Geometry check sheet. Reference: the model listing, model coordinates, mm. A direction names the side the tool comes from. Give positions to 0.01 mm unless a question says otherwise; leave off trailing zeros. One line per item, written item: value.
from build123d import *

# Parameters (mm, degrees)
SKETCH1_W           = 57.15
SKETCH1_H           = 76.2
BOSS_EXTRUDE1_DEPTH = 3.175
CUT_EXTRUDE1_DEPTH  = 1.27


with BuildPart() as part:
    # Sketch1 → Boss-Extrude1 (new body)
    with BuildSketch(Plane(origin=(0, 0, 0), x_dir=(1, 0, 0), z_dir=(0, 1, 0))):
        Rectangle(SKETCH1_W, SKETCH1_H)
    extrude(amount=BOSS_EXTRUDE1_DEPTH)

    # Sketch2 → Cut-Extrude1 (cut)
    # profile 1 of 4: a face of its own
    with BuildSketch(Plane(origin=(0, 3.175, 0), x_dir=(-1, 0, 0), z_dir=(0, 1, 0))):
        with BuildLine():
            Line((6.055318585, -16.590002596), (5.770382688, -16.590002596))
            Line((5.770382688, -16.590002596), (5.770382688, -16.171502996))
            add(Edge.make_bspline(
                [(5.770382688, -16.171502996), (5.740011779, -16.209517079), (5.68116854, -16.283168869), (5.58216602, -16.379210072), (5.478935847, -16.459804005), (5.3698014, -16.523260139), (5.255885696, -16.571252171), (5.137511969, -16.605860082), (5.01403952, -16.626623661), (4.930069938, -16.629335713), (4.88759022, -16.630707724)],
                knots=[0, 0, 0, 0, 1.127869841, 2.185233117, 3.191641716, 4.159226741, 5.10472073, 6.052603964, 7.014823782, 8, 8, 8, 8], degree=3))
            add(Edge.make_bspline(
                [(4.88759022, -16.630707724), (4.844634079, -16.629214017), (4.760516404, -16.626289008), (4.638482352, -16.600515848), (4.523708355, -16.559729658), (4.417729129, -16.502406678), (4.322175382, -16.431236503), (4.239313996, -16.347753357), (4.169631782, -16.252962996), (4.123122139, -16.164236993), (4.093040195, -16.085425579), (4.073271524, -16.0180161), (4.057278247, -15.942883297), (4.04294765, -15.86021293), (4.033387568, -15.769672957), (4.025809426, -15.671479471), (4.020388991, -15.565649476), (4.020173366, -15.492455289), (4.020062175, -15.454711129)],
                knots=[0, 0, 0, 0, 1.235764162, 2.419900973, 3.574701258, 4.732869372, 5.875730734, 6.993815468, 8.107424371, 9.251605764, 9.866123335, 10.534503958, 11.272175692, 12.077112099, 12.949509943, 13.89253218, 14.913238789, 16, 16, 16, 16], degree=3))
            Line((4.020062175, -15.454711129), (4.020062175, -14.269810288))
            Line((4.020062175, -14.269810288), (4.304998072, -14.269810288))
            Line((4.304998072, -14.269810288), (4.304998072, -15.361216538))
            add(Edge.make_bspline(
                [(4.304998072, -15.361216538), (4.305172614, -15.392805516), (4.305506484, -15.453229854), (4.306573304, -15.539742593), (4.30908455, -15.617988608), (4.312758395, -15.688192769), (4.31790085, -15.750098127), (4.323405942, -15.804018032), (4.330082808, -15.849474875), (4.33603676, -15.876838879), (4.338707007, -15.889111169)],
                knots=[0, 0, 0, 0, 1.430803381, 2.736883362, 3.918614142, 4.976458302, 5.92063272, 6.731858525, 7.431260095, 8, 8, 8, 8], degree=3))
            add(Edge.make_bspline(
                [(4.338707007, -15.889111169), (4.348298036, -15.925160767), (4.366708706, -15.994360559), (4.413127221, -16.088064198), (4.470383963, -16.168488135), (4.541323753, -16.233978346), (4.624041324, -16.28496079), (4.718674187, -16.320307963), (4.824242938, -16.342422975), (4.898497037, -16.344624403), (4.937199595, -16.345771826)],
                knots=[0, 0, 0, 0, 1.084232, 2.08126119, 3.027460722, 3.945137793, 4.874029258, 5.839697328, 6.874011781, 8, 8, 8, 8], degree=3))
            add(Edge.make_bspline(
                [(4.937199595, -16.345771826), (4.960123112, -16.345346396), (5.005488159, -16.344504481), (5.072721891, -16.335837862), (5.13814421, -16.32215003), (5.201579846, -16.301932164), (5.263156997, -16.277350064), (5.323130484, -16.247186672), (5.380662305, -16.210701491), (5.436561438, -16.1696921), (5.488517318, -16.124022995), (5.537550393, -16.076530302), (5.580632017, -16.025225386), (5.619738091, -15.971922216), (5.653454407, -15.915550043), (5.682896587, -15.856711455), (5.707874702, -15.79531338), (5.720286952, -15.752700383), (5.726497471, -15.731378798)],
                knots=[0, 0, 0, 0, 1.023939463, 2.026349741, 3.024227553, 4.007104963, 4.997624259, 5.984875705, 7.002218968, 8.038748769, 9.079772093, 10.091408226, 11.086177727, 12.069739863, 13.043026652, 14.017557731, 15.008077027, 16, 16, 16, 16], degree=3))
            add(Edge.make_bspline(
                [(5.726497471, -15.731378798), (5.730071296, -15.715725863), (5.737851324, -15.681650245), (5.746254351, -15.62572995), (5.753881223, -15.561041615), (5.76026475, -15.487660728), (5.764170378, -15.40533037), (5.768428866, -15.314402145), (5.769979229, -15.214513481), (5.770244435, -15.144970374), (5.770382688, -15.10871754)],
                knots=[0, 0, 0, 0, 0.615963638, 1.340920617, 2.168419149, 3.115676021, 4.16674242, 5.331190069, 6.6087489, 8, 8, 8, 8], degree=3))
            Line((5.770382688, -15.10871754), (5.770382688, -14.269810288))
            Line((5.770382688, -14.269810288), (6.055318585, -14.269810288))
            Line((6.055318585, -14.269810288), (6.055318585, -16.590002596))
        make_face()
    # profile 2 of 4: a face of its own
    with BuildSketch(Plane(origin=(0, 3.175, 0), x_dir=(-1, 0, 0), z_dir=(0, 1, 0))):
        with BuildLine():
            Line((1.007882688, -16.590002596), (1.007882688, -14.269810288))
            Line((1.007882688, -14.269810288), (1.292818585, -14.269810288))
            Line((1.292818585, -14.269810288), (1.292818585, -14.671137411))
            add(Edge.make_bspline(
                [(1.292818585, -14.671137411), (1.324992017, -14.63486586), (1.387872244, -14.563976207), (1.491888052, -14.470793448), (1.603055633, -14.394714311), (1.719481041, -14.332960727), (1.842065446, -14.286409707), (1.970088917, -14.25361509), (2.103451285, -14.232281726), (2.194397192, -14.230173515), (2.240484851, -14.22910516)],
                knots=[0, 0, 0, 0, 1.074235403, 2.099501444, 3.086304576, 4.053325556, 5.01427503, 5.985443889, 6.979105517, 8, 8, 8, 8], degree=3))
            add(Edge.make_bspline(
                [(2.240484851, -14.22910516), (2.281458749, -14.23021747), (2.362261091, -14.232410995), (2.481121581, -14.249433739), (2.595511176, -14.276756716), (2.705502779, -14.314802885), (2.810351107, -14.365009415), (2.910646951, -14.425766251), (3.006624386, -14.497409293), (3.09645812, -14.579631484), (3.179287048, -14.668842021), (3.251753995, -14.76427022), (3.313172092, -14.864605375), (3.363646768, -14.969819287), (3.402706719, -15.079835045), (3.429881876, -15.194577175), (3.446886276, -15.313854753), (3.44907869, -15.395080238), (3.45019038, -15.436266618)],
                knots=[0, 0, 0, 0, 1.034036272, 2.039165313, 3.024406509, 3.999331371, 4.971254918, 5.953351348, 6.95522652, 7.989525907, 9.023492927, 10.024309745, 11.009187477, 11.988246066, 12.964946762, 13.950187958, 14.960617622, 16, 16, 16, 16], degree=3))
            add(Edge.make_bspline(
                [(3.45019038, -15.436266618), (3.449054033, -15.476601721), (3.446807536, -15.556342044), (3.430063828, -15.673613807), (3.401929041, -15.78657883), (3.362370202, -15.894818649), (3.311868686, -15.998769181), (3.249394337, -16.097617116), (3.176953503, -16.192874548), (3.093239343, -16.281486741), (3.002599318, -16.363041853), (2.9060849, -16.434859002), (2.804899525, -16.495460062), (2.698840305, -16.544722833), (2.58865823, -16.583870029), (2.473516308, -16.611159395), (2.353938157, -16.627201173), (2.272758349, -16.629527643), (2.231580605, -16.630707724)],
                knots=[0, 0, 0, 0, 1.02050356, 2.017480486, 2.990790918, 3.96161403, 4.928589988, 5.909588639, 6.91611943, 7.952353252, 8.989586576, 9.99823133, 10.991940466, 11.968822692, 12.952985106, 13.945868367, 14.958059758, 16, 16, 16, 16], degree=3))
            add(Edge.make_bspline(
                [(2.231580605, -16.630707724), (2.18422693, -16.629408375), (2.09136861, -16.626860413), (1.955354868, -16.605475308), (1.826625065, -16.569681193), (1.7040642, -16.520825915), (1.589394651, -16.455035241), (1.481514052, -16.373630088), (1.381702446, -16.274636931), (1.322959063, -16.199329814), (1.292818585, -16.160690697)],
                knots=[0, 0, 0, 0, 1.038908319, 2.037250181, 3.012632028, 3.966567879, 4.9252131, 5.905168122, 6.925168603, 8, 8, 8, 8], degree=3))
            Line((1.292818585, -16.160690697), (1.292818585, -16.590002596))
            Line((1.292818585, -16.590002596), (1.007882688, -16.590002596))
        make_face()
        with BuildLine():
            add(Edge.make_bspline(
                [(2.227764499, -16.345771826), (2.269414491, -16.344288631), (2.351624951, -16.34136104), (2.472327468, -16.318543194), (2.587771574, -16.28047983), (2.697769535, -16.228723763), (2.799284509, -16.162425838), (2.891515583, -16.084255444), (2.971962531, -15.993254844), (3.039982689, -15.891514792), (3.096452027, -15.783098406), (3.135420255, -15.668939236), (3.161303129, -15.552122774), (3.163933935, -15.472868592), (3.165254483, -15.43308653)],
                knots=[0, 0, 0, 0, 1.031179624, 2.035384561, 3.030098214, 4.035455833, 5.037557836, 6.024646278, 7.02156144, 8.035264006, 9.049836703, 10.039645228, 11.015989397, 12, 12, 12, 12], degree=3))
            add(Edge.make_bspline(
                [(3.165254483, -15.43308653), (3.163540249, -15.393551932), (3.160118502, -15.3146377), (3.136215415, -15.197642221), (3.094258569, -15.08422785), (3.039024474, -14.974413926), (2.969933592, -14.871915003), (2.889645422, -14.779234125), (2.79694635, -14.699858737), (2.694537475, -14.633373426), (2.585275386, -14.579891334), (2.47033249, -14.542170246), (2.351712204, -14.518353481), (2.270912571, -14.515483367), (2.230308569, -14.514041057)],
                knots=[0, 0, 0, 0, 0.979235476, 1.954632679, 2.943119654, 3.967171814, 4.992637064, 5.997548408, 6.995574264, 8.005058949, 9.015076297, 9.999929117, 10.994910263, 12, 12, 12, 12], degree=3))
            add(Edge.make_bspline(
                [(2.230308569, -14.514041057), (2.189082755, -14.51554163), (2.107297234, -14.51851853), (1.986177363, -14.541493739), (1.868854415, -14.580029732), (1.756283853, -14.632504372), (1.651593001, -14.697560163), (1.558068615, -14.774059954), (1.477272541, -14.861666513), (1.41075029, -14.959856368), (1.357599909, -15.066314478), (1.319965408, -15.180022076), (1.297107538, -15.300303471), (1.294268004, -15.382739468), (1.292818585, -15.424818301)],
                knots=[0, 0, 0, 0, 1.017730373, 2.019016736, 3.032373701, 4.060729657, 5.079187105, 6.068726676, 7.03591854, 8.011858086, 8.988317194, 9.965225429, 10.961364673, 12, 12, 12, 12], degree=3))
            add(Edge.make_bspline(
                [(1.292818585, -15.424818301), (1.293689144, -15.456874749), (1.29540268, -15.519971983), (1.308493072, -15.612616408), (1.329317189, -15.701274213), (1.358657167, -15.786042436), (1.397212571, -15.8664383), (1.443664912, -15.943091998), (1.498966997, -16.015289511), (1.561435842, -16.082939407), (1.630584648, -16.14433424), (1.704115441, -16.198447131), (1.781843219, -16.244241527), (1.863713421, -16.280889022), (1.949095477, -16.310744817), (2.038807758, -16.330464053), (2.131946128, -16.344047564), (2.195488753, -16.345191021), (2.227764499, -16.345771826)],
                knots=[0, 0, 0, 0, 1.050062701, 2.066855696, 3.059271411, 4.030305351, 4.999747758, 5.975466543, 6.961907836, 7.974539719, 8.98812422, 9.98710676, 10.961662635, 11.93785114, 12.922015094, 13.919620009, 14.94329489, 16, 16, 16, 16], degree=3))
        make_face(mode=Mode.SUBTRACT)
    # profile 3 of 4: a face of its own
    with BuildSketch(Plane(origin=(0, 3.175, 0), x_dir=(-1, 0, 0), z_dir=(0, 1, 0))):
        Polygon((0.600831406, -16.590002596), (0.292362856, -16.590002596), (-0.477854492, -14.900739775), (-1.248071839, -16.590002596), (-1.556540389, -16.590002596), (-0.498207056, -14.269810288), (-0.457501928, -14.269810288), align=None)
    # profile 4 of 4: a face of its own
    with BuildSketch(Plane(origin=(0, 3.175, 0), x_dir=(-1, 0, 0), z_dir=(0, 1, 0))):
        Polygon((-1.943239107, -17.444810288), (-2.272060221, -17.444810288), (-3.103335261, -16.146062291), (-3.934610301, -17.444810288), (-4.263431415, -17.444810288), (-3.268063827, -15.889111169), (-4.304136543, -14.269810288), (-3.975315429, -14.269810288), (-3.103335261, -15.632160048), (-2.231355093, -14.269810288), (-1.902533979, -14.269810288), (-2.939242713, -15.889111169), align=None)
    extrude(amount=-CUT_EXTRUDE1_DEPTH, mode=Mode.SUBTRACT)


solid = part.part
1) Mould release check, pull along X, two halves, no side actions. Record for faces 3 (the flat face through (3.1, 1.905, -15.8)), 4 (the flat face through (0, 2, 38.1)), 5 (the flat face through (28.575, 2, 1)): released by +X, released by -X, zero draft, split by the parting line, or undercut.
Verdict:
face 3: undercut
face 4: zero draft
face 5: released by +X
2) Tool access check on faces 1 (the flat face through (0, 3.175, -1)), 2 (the flat face through (-1.16, 1.905, -15.68)). Record the directions out of +Z, -Z, +X, -X, +Y, -Y that give a thin tool (end or side, any length) a straight path to the whole face; none if there is none.
Verdict:
face 1: +Z, -Z, +X, -X, +Y
face 2: +Y
3) Scan line: probe 1 along Z at (x, y) = (0, 2.85). Record every from-to range of solid material in increasing order.
Verdict:
probe 1: -38.1 to -15.95, -15.27 to 38.1
